Geometry check sheet. Reference: drawing and pictorial views, mm from the part's lowest x, y, z. A direction names the side the tool comes from. Round coordinates to 2 decimals unless told otherwise and drop trailing zeros. Write each loop counter-clockwise with the first axis right and the second up, starting at its lowest first coordinate (ties: lowest second). Pieces come first, ordered by that corner, then holes. Notation, with made-up numbers: M 21,5.5 L 44,5.5 A22 cw 44,31.5 Z; hole C 23,14.5 d2. An arc over 180 degrees is marked long. One line per question, with ' | ' between items.
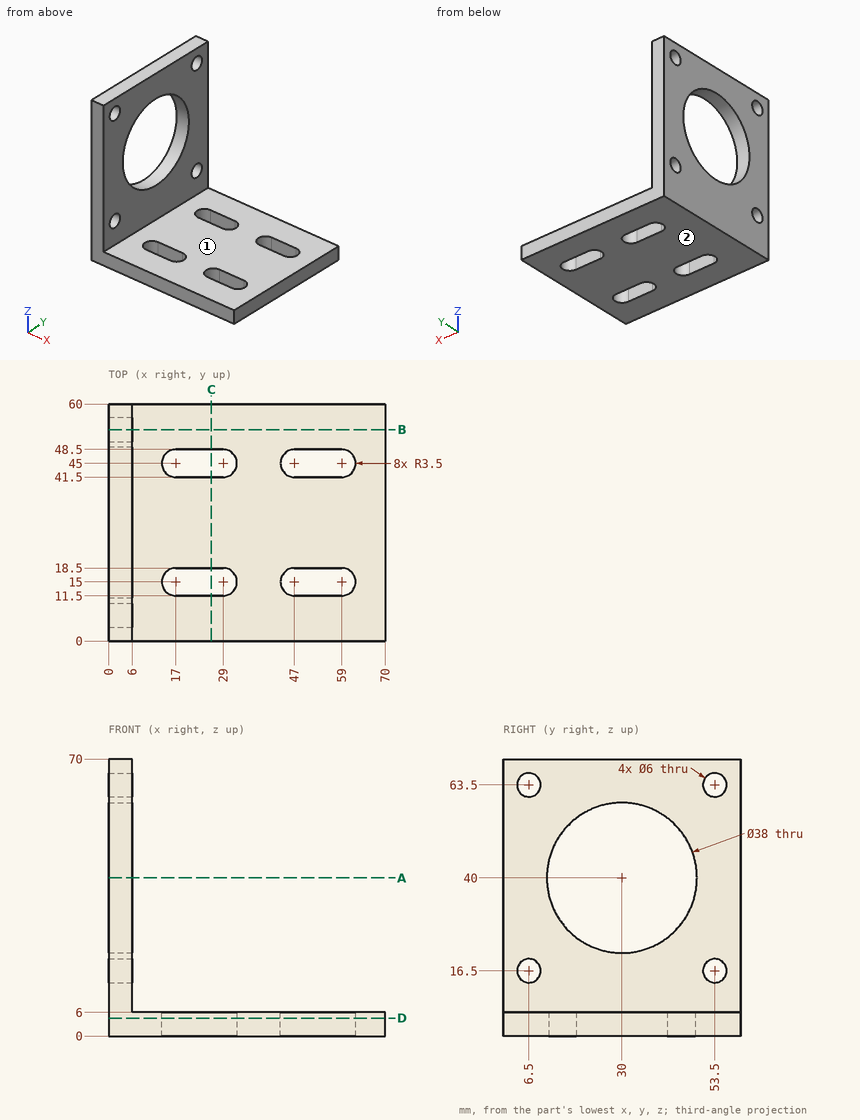
1. Section check A-A, the plane z = 40. Record the cut outline in (x, y).
Results:
outline: M 0,0 L 6,0 L 6,11 L 0,11 Z; M 0,49 L 6,49 L 6,60 L 0,60 Z
2. Section check D-D, the plane z = 4.5. Record the cut outline in (x, y), then the cut area to 3 significant figures.
Results:
outline: M 0,0 L 70,0 L 70,60 L 0,60 Z; hole M 17,11.5 L 29,11.5 A3.5 ccw 29,18.5 L 17,18.5 A3.5 ccw Z; hole M 17,41.5 L 29,41.5 A3.5 ccw 29,48.5 L 17,48.5 A3.5 ccw Z; hole M 47,11.5 L 59,11.5 A3.5 ccw 59,18.5 L 47,18.5 A3.5 ccw Z; hole M 47,41.5 L 59,41.5 A3.5 ccw 59,48.5 L 47,48.5 A3.5 ccw Z | area: 3,710 mm2
3. Tool access check on the marked faces 1 and 2. Record the directions out of +Z, -Z, +X, -X, +Y, -Y that give a thin tool (end or side, any length) a straight path to the whole face; none if there is none.
Results:
face 1: +Z, +X, +Y, -Y | face 2: -Z, +X, -X, +Y, -Y
4. Section check B-B, the plane y = 53.5. Record the cut outline in (x, z), then the cut area to 3 significant figures.
Results:
outline: M 0,0 L 70,0 L 70,6 L 6,6 L 6,13.5 L 0,13.5 Z; M 0,19.5 L 6,19.5 L 6,60.5 L 0,60.5 Z; M 0,66.5 L 6,66.5 L 6,70 L 0,70 Z | area: 732 mm2
5. Thickness scan on line 1 (Z direction, x = 1.85, y = 53.5); line 2 (Y direction, x = 1, z = 63); line 3 (X direction, y = 4, z = 36). Record the ranges inside material, lowest first.
Results:
line 1: z = 0 to 13.5, 19.5 to 60.5, 66.5 to 70 | line 2: y = 0 to 3.54, 9.46 to 50.54, 56.46 to 60 | line 3: x = 0 to 6
6. Go/stop test with flat-tipped pins: P1, Ø1.5, axis at y = 11, z = 50, coming from the -X side; P2, Ø23, axis at y = 30, z = 40, coming from the +X side; P3, Ø8, axis at x = 11, y = 44.5, coming from the +Z side; P4, Ø18, axis at y = 18.5, z = 49.5, coming from the +X side. Record where each tip stops, or that it passes through.
Results:
P1: stops at x = 0 | P2: passes through | P3: stops at z = 6 | P4: stops at x = 6
7. Section check C-C, the plane x = 26. Record the cut outline in (y, z), then the cut area to 3 significant figures.
Results:
outline: M 0,0 L 11.5,0 L 11.5,6 L 0,6 Z; M 18.5,0 L 41.5,0 L 41.5,6 L 18.5,6 Z; M 48.5,0 L 60,0 L 60,6 L 48.5,6 Z | area: 276 mm2
